Work out the finished part from the listing and answer in its coordinate system (mm). Face numbers are marked on the shaded views. A direction names the side the tool comes from. Give positions to 0.01 mm unless a question says otherwise; leave off trailing zeros. Order: outer loops, then holes, each group sorted by start corner. A loop starts at its lowest first (then second) coordinate and runs counter-clockwise, first axis right, second up. Notation, with made-up numbers: M 64,-8 L 96,-8 A9 cw 96,-3 Z; hole C 20.25,5.25 d7. An arc over 180 degrees is marked long. One line per item, written item: value.
from build123d import *

# Parameters (mm, degrees)
SKETCH1_R           = 0.75
BOSS_EXTRUDE1_DEPTH = 10
FILLET1_R           = 3
FILLET2_R           = 5
SKETCH2_R           = 1.5
CUT_EXTRUDE1_DEPTH  = 10


# Read off the part's stored shape, not the designer's step: Mirror10
with BuildPart() as part:
    # Sketch1 → Boss-Extrude1 (new body)
    with BuildSketch(Plane(origin=(0, 0, 0), x_dir=(0, 0, -1), z_dir=(1, 0, 0))):
        with BuildLine():
            Line((5.15, 0), (15.15, 0))
            Line((15.15, 0), (15.15, 50))
            Line((15.15, 50), (0.05, 50))
            Line((0.05, 50), (0.05, 41.5))
            ThreePointArc((0.05, 41.5), (1.55, 40), (0.05, 38.5))
            Line((0.05, 38.5), (0.05, 26.5))
            ThreePointArc((0.05, 26.5), (1.55, 25), (0.05, 23.5))
            Line((0.05, 23.5), (0.05, 10))
            Line((0.05, 10), (5.15, 10))
            Line((5.15, 10), (5.15, 0))
        make_face()
        with Locations((2.55, 15)):
            Circle(SKETCH1_R, mode=Mode.SUBTRACT)
    extrude(amount=BOSS_EXTRUDE1_DEPTH)

    # Fillet1
    fillet1_edges = [part.edges().sort_by_distance(p)[0] for p in [
        (5, 0, -15.15),
        (10, 0, -10.15),
        (10, 25, -15.15),
        (10, 50, -7.6),
    ]]
    fillet(fillet1_edges, radius=FILLET1_R)

    # Fillet2
    # the kernel refuses this fillet: 5 mm, written as the material it takes off along each edge
    with BuildSketch(Plane(origin=(0, 10, 12.45), x_dir=(0, 1, 0), z_dir=(0, 0, -1))) as fillet2_piece_1:
        with BuildLine():
            CenterArc((FILLET2_R, FILLET2_R), FILLET2_R, 180, 90)
            Line((0, FILLET2_R), (0, 0))
            Line((0, 0), (FILLET2_R, 0))
        make_face()
    extrude(amount=17.6, mode=Mode.SUBTRACT)
    with BuildSketch(Plane(origin=(10, 10, 12.45), x_dir=(0, 1, 0), z_dir=(0, 0, -1))) as fillet2_piece_2:
        with BuildLine():
            CenterArc((FILLET2_R, -FILLET2_R), FILLET2_R, 90, 90)
            Line((0, -FILLET2_R), (0, 0))
            Line((0, 0), (FILLET2_R, 0))
        make_face()
    extrude(amount=17.6, mode=Mode.SUBTRACT)

    # Sketch2 → Cut-Extrude1 (cut)
    with BuildSketch(Plane(origin=(0, 0, -15.15), x_dir=(-1, 0, 0), z_dir=(0, 0, -1))):
        with Locations((-5, 5)):
            Circle(SKETCH2_R)
    extrude(amount=-CUT_EXTRUDE1_DEPTH, mode=Mode.SUBTRACT)

    # Mirror10: part across plane


with BuildPart() as part_1:
    add(part.part)
    add(part.part.mirror(Plane(origin=(10, 50, -0.05), x_dir=(1, 0, 0), z_dir=(0, 0, -1))))


solid = part_1.part
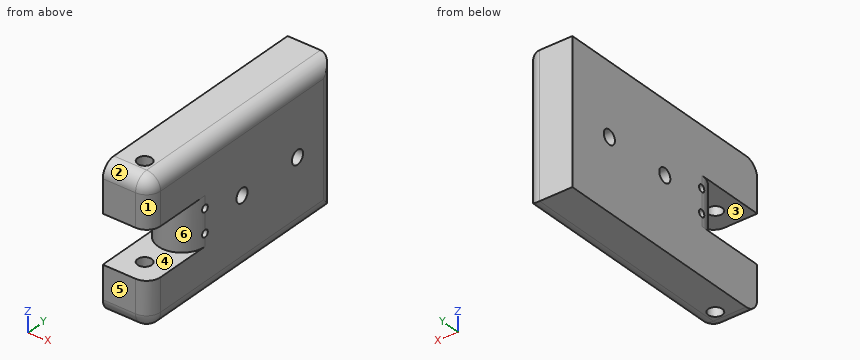
(1) Determine the mould class of the marked faces 1, 2, 3 and 4 for opening direction Z: pulls with the +Z half, pulls with the -Z half, needs draft (parallel to the pull), parting line crosses it, or undercut.
Findings:
face 1: needs draft
face 2: pulls with the +Z half
face 3: undercut
face 4: undercut
(2) Find the intervals of material crossed by probe 1 along Z at (x, y) = (7.25, 15); probe 2 along Z at (x, y) = (5, 15); probe 3 along Z at (x, y) = (2, 40), in increasing order. Write a range as from..to.
Findings:
probe 1: z = -15.14..-3.3, -1.8..1.7, 3.2..15.04
probe 2: z = -15.15..-3.3, -1.8..1.7, 3.2..15.05
probe 3: z = -15.15..-1.55, 1.45..15.05
(3) Section B-B, the plane y = 5 is taken. Give the vertices of the cut face in (x, z).
Findings:
outline: M 0,-15.15 L 3.5,-15.15 L 3.5,-5.15 L 0,-5.15 Z; M 0,5.05 L 3.5,5.05 L 3.5,15.05 L 0,15.05 Z; M 6.5,-15.15 L 7,-15.15 A3 ccw 10,-12.15 L 10,-5.15 L 6.5,-5.15 Z; M 6.5,5.05 L 10,5.05 L 10,12.05 A3 ccw 7,15.05 L 6.5,15.05 Z
(4) Section D-D, the plane y = 40 is taken. Give the vertices of the cut face in (x, z).
Findings:
outline: M 0,-15.15 L 7,-15.15 A3 ccw 10,-12.15 L 10,-1.55 L 0,-1.55 Z; M 0,1.45 L 10,1.45 L 10,12.05 A3 ccw 7,15.05 L 0,15.05 Z
(5) Which of the six approach directions +Z, -Z, +X, -X, +Y, -Y give full straight-line access (tool end or side, diameter ignored) to the marked faces 5 and 6?
Findings:
face 5: +Z, -Z, +X, -X, -Y
face 6: -Y
(6) Section A-A, the plane x = 5 is taken. Give the vertices of the cut face in (y, z), then the cut area to 3 significant figures.
Findings:
outline: M 0,-12.15 A3 ccw 3,-15.15 L 3.5,-15.15 L 3.5,-5.15 L 0,-5.15 Z; M 0,5.05 L 3.5,5.05 L 3.5,15.05 L 3,15.05 A3 ccw 0,12.05 Z; M 6.5,-15.15 L 50,-15.15 L 50,15.05 L 6.5,15.05 L 6.5,5.05 L 10,5.05 L 10,-5.15 L 6.5,-5.15 Z; hole C 15,-2.55 d1.5; hole C 15,2.45 d1.5; hole C 25,-0.05 d3; hole C 40,-0.05 d3
area: 1,330 mm^2
(7) Section C-C, the plane z = -2.55 is taken. Give the vertices of the cut face in (x, y), then the cut area to 3 significant figures.
Findings:
outline: M 0,15.75 L 10,15.75 L 10,47 A3 ccw 7,50 L 0,50 Z; M 0.06,14.25 A5 ccw 9.94,14.25 Z
area: 372 mm^2
